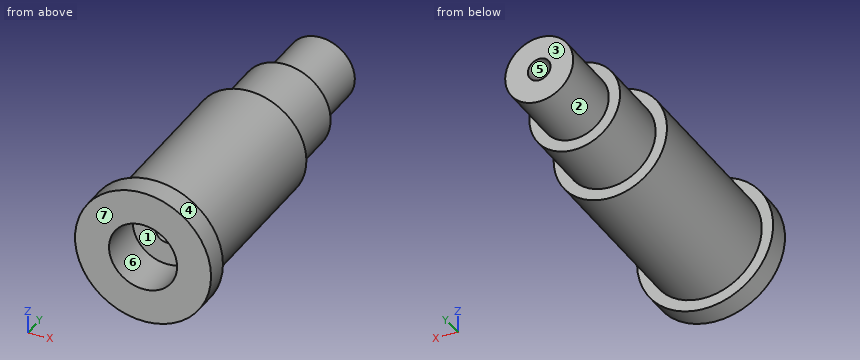
```python
from build123d import *

# Parameters (mm, degrees)
F0_R     = 3
F1_DEPTH = 15
F2_R     = 1.5
F3_DEPTH = 2
F4_W     = 5.878874
F4_H     = 2.213873
F6_R     = 0.5
F7_DEPTH = 13.001
F8_W     = 16.149964
F8_H     = 2.257945
F10_W    = 4.508098
F10_H    = 1.941308


with BuildPart() as f1:
    # F0 (on Front) → F1 (new body)
    with BuildSketch(Plane.XZ):
        Circle(F0_R)
    extrude(amount=F1_DEPTH)

    # F2 (on face) → F3 (cut)
    with BuildSketch(Plane.XZ.offset(15)):
        Circle(F2_R)
    extrude(amount=-F3_DEPTH, mode=Mode.SUBTRACT)

    # F4 (on Right) → F5 (revolve, cut)
    with BuildSketch(Plane.YZ):
        with Locations((-0.060563, 2.606936)):
            Rectangle(F4_W, F4_H)
    revolve(axis=Axis((0, -8.455116, 0), (0, 1, 0)), mode=Mode.SUBTRACT)

    # F6 (on face) → F7 (cut, through all)
    with BuildSketch(Plane.XZ.offset(13)):
        Circle(F6_R)
    extrude(amount=-F7_DEPTH, mode=Mode.SUBTRACT)

    # F8 (on Right) → F9 (revolve, cut)
    with BuildSketch(Plane.YZ):
        with Locations((-5.925018, 3.628972)):
            Rectangle(F8_W, F8_H)
    revolve(axis=Axis((0, -7.437502, 0), (0, 1, 0)), mode=Mode.SUBTRACT)

    # F10 (on Right) → F11 (revolve, cut)
    with BuildSketch(Plane.YZ):
        with Locations((-3.745951, 2.970654)):
            Rectangle(F10_W, F10_H)
    revolve(axis=Axis((0, -6.562206, 0), (0, 1, 0)), mode=Mode.SUBTRACT)


solid = f1.part
```
The model under review builds one solid part; all positions refer to its coordinate system, in mm. Face numbers are marked on the shaded views. A direction names the side the tool comes from. Round coordinates to 2 decimals unless told otherwise and drop trailing zeros. Loops run counter-clockwise (first coordinate to the right, second up) from the corner with the lowest first, then second, coordinate; pieces in that order, holes last. Notation, with made-up numbers: M 9,63.5 L 30,63.5 A34 cw 30,100.5 Z; hole C 6,-40 d4. An arc over 180 degrees is marked long. Write item = value, one per line.
Item 1: Insertion check: P1, Ø3, axis at y = -3, z = -0.5, coming from the -X side; P2, Ø0.9, axis at x = -0.5, z = -0.5, coming from the -Y side. Each pin has a flat end and moves straight along its axis. Give the tip position at first contact, or say it passes through.
Return value:
P1 = -2
P2 = -13
Item 2: Take a section at A-A on x = 0. Write out the cut boundary in (y, z).
Return value:
outline = M -15,-3 L -14,-3 L -14,-2.5 L -6,-2.5 L -6,-2 L -3,-2 L -3,-1.5 L 0,-1.5 L 0,-0.5 L -13,-0.5 L -13,-1.5 L -15,-1.5 Z; M -15,1.5 L -13,1.5 L -13,0.5 L 0,0.5 L 0,1.5 L -3,1.5 L -3,2 L -6,2 L -6,2.5 L -14,2.5 L -14,3 L -15,3 Z
Item 3: For line 1 (Z direction, x = 0, y = -14.6); line 2 (Y direction, x = 0.4, z = -1.85); line 3 (Y direction, x = -2.55, z = -0.2), list the stretches that pass through material, from the lowest coordinate up. Write a range as [from, to].
Return value:
line_1 = [-3, -1.5], [1.5, 3]
line_2 = [-15, -3]
line_3 = [-15, -14]
Item 4: Take a section at B-B on z = 0. Write out the cut boundary in (x, y).
Return value:
outline = M -3,-15 L -1.5,-15 L -1.5,-13 L -0.5,-13 L -0.5,0 L -1.5,0 L -1.5,-3 L -2,-3 L -2,-6 L -2.5,-6 L -2.5,-14 L -3,-14 Z; M 0.5,-13 L 1.5,-13 L 1.5,-15 L 3,-15 L 3,-14 L 2.5,-14 L 2.5,-6 L 2,-6 L 2,-3 L 1.5,-3 L 1.5,0 L 0.5,0 Z
Item 5: Machinability: for the marked faces 1, 2 and 3, which of the approach directions +Z, -Z, +X, -X, +Y, -Y give a long, thin tool a straight path to every point of the face, cutting with its end or side? Answer none if there is none.
Return value:
face_1 = -Y
face_2 = +Y
face_3 = +Z, -Z, +X, -X, +Y
Item 6: Take a section at D-D on y = -8.25. Write out the cut boundary in (x, z), then the cut area to 3 significant figures.
Return value:
outline = C 0,0 d5; hole C 0,0 d1
area = 18.8 mm2
Item 7: The part is to be moulded in two halves that separate along Z. For the marked faces 4, 5, 6 and 7, say which applies: released by +Z, released by -Z, zero draft, split by the parting line, or undercut.
Return value:
face_4 = split by the parting line
face_5 = undercut
face_6 = undercut
face_7 = zero draft
Item 8: Take a section at C-C on x = -2.3. Write out the cut boundary in (y, z).
Return value:
outline = M -15,-1.93 L -14,-1.93 L -14,-0.98 L -6,-0.98 L -6,0.98 L -14,0.98 L -14,1.93 L -15,1.93 Z
